```python
from build123d import *

# Parameters (mm, degrees)
SKETCH1_W           = 41.9
SKETCH1_H           = 21
SKETCH1_R           = 1.25
SKETCH1_R_2         = 1.5
SKETCH1_R_3         = 4
BOSS_EXTRUDE1_DEPTH = 2
SKETCH1_3_W         = 2
SKETCH1_3_H         = 21
BOSS_EXTRUDE2_DEPTH = 31.31
SKETCH2_R           = 1.5
CUT_EXTRUDE1_DEPTH  = 50
FILLET1_R           = 1


with BuildPart() as part:
    # Sketch1 → Boss-Extrude1 (new body)
    with BuildSketch(Plane.XY):
        Rectangle(SKETCH1_W, SKETCH1_H)
        with Locations((-6, -8)):
            Circle(SKETCH1_R, mode=Mode.SUBTRACT)
        with Locations((6, -8)):
            Circle(SKETCH1_R, mode=Mode.SUBTRACT)
        with Locations((0, -7)):
            Circle(SKETCH1_R_2, mode=Mode.SUBTRACT)
        Circle(SKETCH1_R_3, mode=Mode.SUBTRACT)
        with Locations((7, 0)):
            Circle(SKETCH1_R_2, mode=Mode.SUBTRACT)
        with Locations((-7, 0)):
            Circle(SKETCH1_R_2, mode=Mode.SUBTRACT)
        with Locations((-6, 8)):
            Circle(SKETCH1_R, mode=Mode.SUBTRACT)
        with Locations((0, 7)):
            Circle(SKETCH1_R_2, mode=Mode.SUBTRACT)
        with Locations((6, 8)):
            Circle(SKETCH1_R, mode=Mode.SUBTRACT)
    extrude(amount=BOSS_EXTRUDE1_DEPTH)

    # Sketch1_3 → Boss-Extrude2 (add)
    with BuildSketch(Plane.XY):
        with Locations((-21.95, 0)):
            Rectangle(SKETCH1_3_W, SKETCH1_3_H)
        with Locations((21.95, 0)):
            Rectangle(SKETCH1_3_W, SKETCH1_3_H)
    extrude(amount=BOSS_EXTRUDE2_DEPTH)

    # Sketch2 → Cut-Extrude1 (cut)
    with BuildSketch(Plane.ZY.offset(22.95)):
        with Locations(Location((16.55, 0, 0), (0, 0, 180))):
            Circle(SKETCH2_R)
        with BuildLine():
            Line((31.31, 10.5), (23.55, 10.5))
            ThreePointArc((23.55, 10.5), (27.791446457, 9.60521379), (31.31, 7.073358467))
            Line((31.31, 7.073358467), (31.31, 10.5))
        make_face()
        with BuildLine():
            ThreePointArc((31.31, -7.073358467), (27.791446457, -9.60521379), (23.55, -10.5))
            Line((23.55, -10.5), (31.31, -10.5))
            Line((31.31, -10.5), (31.31, -7.073358467))
        make_face()
        with Locations(Location((23.55, 7, 0), (0, 0, 180))):
            Circle(SKETCH2_R)
        with Locations(Location((23.55, -7, 0), (0, 0, 180))):
            Circle(SKETCH2_R)
        with BuildLine():
            Line((31.31, -4.25), (31.31, 4.25))
            Line((31.31, 4.25), (23.55, 4.25))
            ThreePointArc((23.55, 4.25), (19.3, 0), (23.55, -4.25))
            Line((23.55, -4.25), (31.31, -4.25))
        make_face()
    extrude(amount=-CUT_EXTRUDE1_DEPTH, mode=Mode.SUBTRACT)

    # Fillet1
    fillet1_edges = [part.edges().sort_by_distance(p)[0] for p in [
        (-22.95, 0, 0),
        (22.95, 0, 0),
    ]]
    fillet(fillet1_edges, radius=FILLET1_R)


solid = part.part
```
The listing builds one solid part. Answer for the finished solid, in the listing's coordinates (mm). A direction names the side the tool comes from. Coordinates: 2 decimals unless noted, no trailing zeros. Write each loop counter-clockwise with the first axis right and the second up, starting at its lowest first coordinate (ties: lowest second). Pieces come first, ordered by that corner, then holes. Notation, with made-up numbers: (-2.5, 8) -> (54.5, 8) arc R25 ccw to (54.5, 37) -> close; hole circle Ø4 at (-36, 52.5). An arc over 180 degrees is marked (long way). Write each question's results on one line, items separated by ' | '. Start each with the question number.
1) Flat-ended cylindrical pins translate along their axes: pin 1 Ø4 at (x, y) = (-6, 8) entering from +Z; pin 2 Ø4 at (y, z) = (7, 23.55) entering from -X; pin 3 Ø2 at (x, z) = (-22.5, 26) entering from +Y; pin 4 Ø0.6 at (x, z) = (22, 29.5) entering from +Y. Find the tip coordinate at first contact, or state that the pin passes through.
2) Straight lines are drawn through the part: probe 1 along Y at (x, z) = (0, 0.85); probe 2 along Y at (x, z) = (-22.05, 23.55); probe 3 along X at (y, z) = (-5.5, 17). For each, find the intervals that lie inside material, in ascending order.
3) A cutting plane is placed at A-A (x = 0). Determine the outline of the cut face in (y, z), then the cut area to 3 significant figures.
4) A cutting plane is placed at C-C (z = 16.55). Determine the outline of the cut face in (x, y).
5) A tool of negligible diameter and unlimited length cuts with its end or side. For faces 1 (the flat face through (4.4, 0.1, 2)), 2 (the cylindrical face through (-21.96, 7.91, 24.74)), from which of +Z, -Z, +X, -X, +Y, -Y can it reach the whole face along a straight path? Write none if from no direction.
6) A cutting plane is placed at B-B (y = 0). Count the separate pieces of the cut face and the enclosed holes in it, then the cut area to 3 significant figures.
7) For a pull along Z with two mould halves and no side action, classify faces 3 (the cylindrical face through (5.01, -8.76, 0.99)), 4 (the cylindrical face through (22.649, 0.147, 0.285)), 5 (the cylindrical face through (21.94, -0.07, 18.05)), 6 (the flat face through (22, 6, 31.31)) as +Z half, -Z half, draft (parallel to the pull), parting line (faces both ways), or undercut.
Values follow:
1) pin 1: z = 2 | pin 2: x = -22.95 | pin 3: y = 10.4 | pin 4: y = 8.85
2) probe 1: -10.5 to -8.5, -5.5 to -4, 4 to 5.5, 8.5 to 10.5 | probe 2: -10.5 to -8.5, -5.5 to -4.25, 4.25 to 5.5, 8.5 to 10.5 | probe 3: -22.95 to -20.95, 20.95 to 22.95
3) outline: (-10.5, 0) -> (-8.5, 0) -> (-8.5, 2) -> (-10.5, 2) -> close; (-5.5, 0) -> (-4, 0) -> (-4, 2) -> (-5.5, 2) -> close; (4, 0) -> (5.5, 0) -> (5.5, 2) -> (4, 2) -> close; (8.5, 0) -> (10.5, 0) -> (10.5, 2) -> (8.5, 2) -> close | area: 14.0 mm²
4) outline: (-22.95, -10.5) -> (-20.95, -10.5) -> (-20.95, -1.5) -> (-22.95, -1.5) -> close; (-22.95, 1.5) -> (-20.95, 1.5) -> (-20.95, 10.5) -> (-22.95, 10.5) -> close; (20.95, -10.5) -> (22.95, -10.5) -> (22.95, -1.5) -> (20.95, -1.5) -> close; (20.95, 1.5) -> (22.95, 1.5) -> (22.95, 10.5) -> (20.95, 10.5) -> close
5) face 1: +Z, +Y, -Y | face 2: +X, -X
6) separate pieces: 6 | enclosed holes: 0 | area: 121 mm²
7) face 3: draft | face 4: -Z half | face 5: undercut | face 6: +Z half
